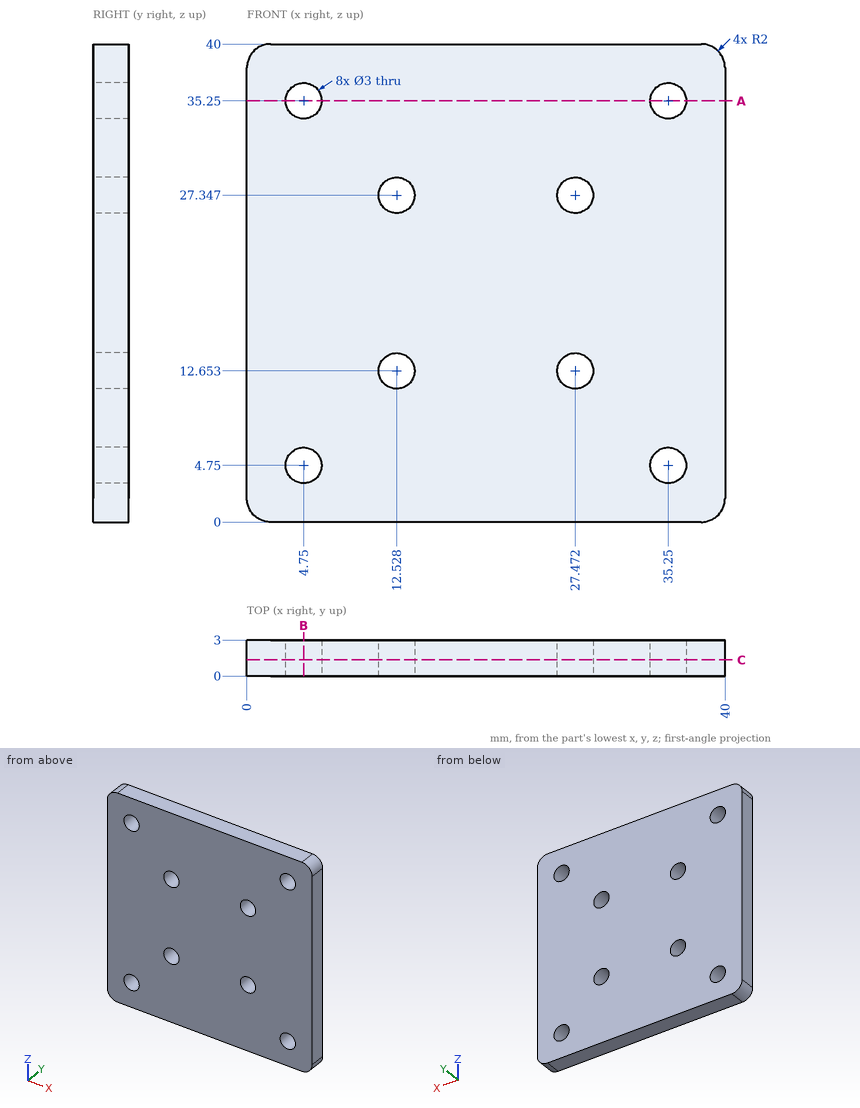
Check sheet for the drawn part. Datum: minimum x, y, z corner. Units: mm. Give positions to 0.01 mm unless a question says otherwise; leave off trailing zeros. Order: outer loops, then holes, each group sorted by start corner. A loop starts at its lowest first (then second) coordinate and runs counter-clockwise, first axis right, second up. Notation, with made-up numbers: (-30, -29) - (-16, -29) arc R19 ccw to (-16, -19) - close; hole circle Ø4 at (54.25, 17.5). An arc over 180 degrees is marked (long way). Answer as a JSON object with one key per item and string values.
(1) Cross-section at B-B (x = 4.75). Record the cut outline in (y, z), then the cut area to 3 significant figures.
Report:
{"outline": "(0, 0) - (3, 0) - (3, 3.25) - (0, 3.25) - close; (0, 6.25) - (3, 6.25) - (3, 33.75) - (0, 33.75) - close; (0, 36.75) - (3, 36.75) - (3, 40) - (0, 40) - close", "area": "102 mm^2"}
(2) Cross-section at A-A (z = 35.25). Record the cut outline in (x, y).
Report:
{"outline": "(0, 0) - (3.25, 0) - (3.25, 3) - (0, 3) - close; (6.25, 0) - (33.75, 0) - (33.75, 3) - (6.25, 3) - close; (36.75, 0) - (40, 0) - (40, 3) - (36.75, 3) - close"}
(3) Material ranges on line 1 (Z direction, x = 35.25, y = 2.2); line 2 (X direction, y = 1.55, z = 34); line 3 (Z direction, x = 27, y = 2.6), recorded low to high.
Report:
{"line 1": "0 to 3.25, 6.25 to 33.75, 36.75 to 40", "line 2": "0 to 3.92, 5.58 to 34.42, 36.08 to 40", "line 3": "0 to 11.23, 14.08 to 25.92, 28.77 to 40"}
(4) Cross-section at C-C (y = 1.35). State how many separate pieces and enclosed holes the cut face has, then the cut area to 3 significant figures.
Report:
{"separate pieces": "1", "enclosed holes": "8", "area": "1,540 mm^2"}
